Input: dimensioned drawing with shaded views. Units: mm. Origin: part minimum x, y, z. Round coordinates to 2 decimals unless told otherwise and drop trailing zeros. Write each loop counter-clockwise with the first axis right and the second up, starting at its lowest first coordinate (ties: lowest second). Pieces come first, ordered by that corner, then holes. Notation, with made-up numbers: (53, 19) -> (68, 19) arc R27 cw to (68, 57) -> close; hole circle Ø7 at (25, 15.5). An arc over 180 degrees is marked (long way). One line per item, written item: value. Start each with the question number.
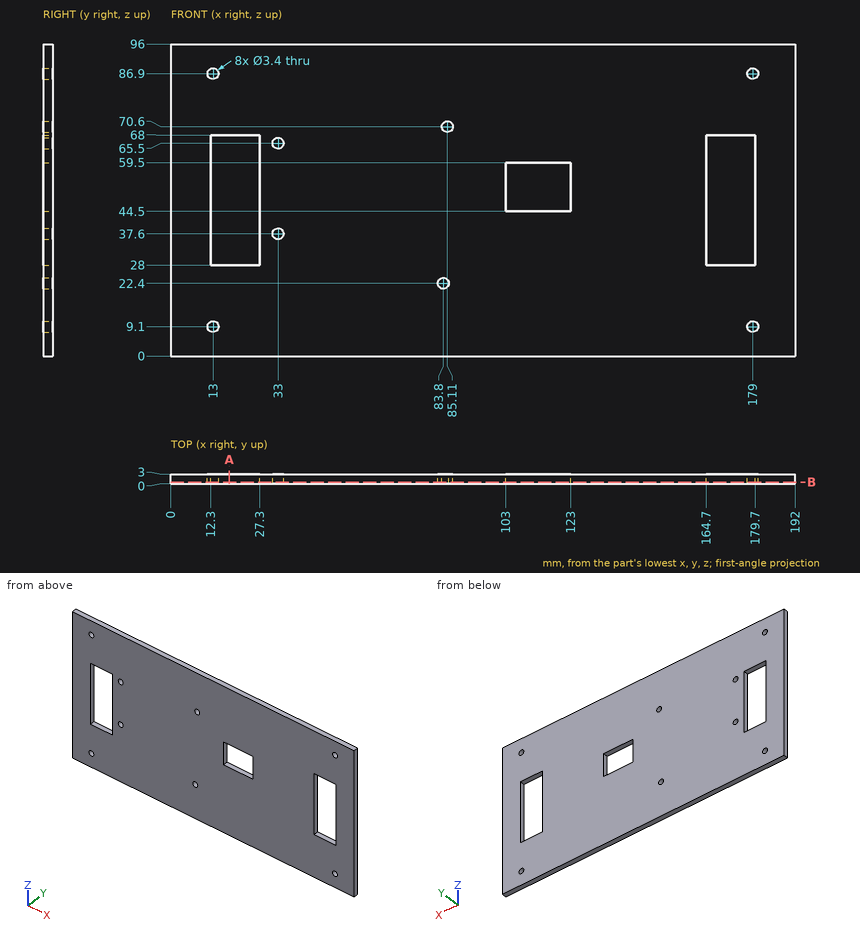
(1) Section query A-A (x = 18). Output: boundary loops of the cut face in (y, z).
(2) Section query B-B (y = 0.55). Count the separate pieces of the cut face and the enclosed holes in it, and give its area (3 significant figures).
(3) Line query: probe 1 along X at (y, z) = (2.1, 56); probe 2 along X at (y, z) = (1.9, 9.1); probe 3 along Z at (x, y) = (13, 2.1). Output: solid intervals per line, ascending.
Results list:
1. outline: (0, 0) -> (3, 0) -> (3, 28) -> (0, 28) -> close; (0, 68) -> (3, 68) -> (3, 96) -> (0, 96) -> close
2. separate pieces: 1
2. enclosed holes: 11
2. area: 16,900 mm^2
3. probe 1: x = 0 to 12.3, 27.3 to 103, 123 to 164.7, 179.7 to 192
3. probe 2: x = 0 to 11.3, 14.7 to 177.3, 180.7 to 192
3. probe 3: z = 0 to 7.4, 10.8 to 28, 68 to 85.2, 88.6 to 96
